Part model, mm, in its own coordinate system. Face numbers are marked on the shaded views. A direction names the side the tool comes from. Round coordinates to 2 decimals unless told otherwise and drop trailing zeros. Loops run counter-clockwise (first coordinate to the right, second up) from the corner with the lowest first, then second, coordinate; pieces in that order, holes last. Notation, with made-up numbers: M 18,29.25 L 57,29.25 A17 ccw 57,44.25 Z; hole C 40.5,34.5 d5. An arc over 180 degrees is marked long. Answer as CSV lines item,"result". Start each with the question number.
Item 1: Which spindle directions (+Z, -Z, +X, -X, +Y, -Y) get a long thin tool onto all of the face, cutting with end or side? Do the marked faces 1 and 2. Say none if no direction does.
Item 2: Band-saw the part on B-B (x = 14.5). Give the cut face in (y, z), and give its area (3 significant figures).
Item 3: Drop flat-ended pins along their axis: pin 1 Ø8 at (y, z) = (0, 0) entering from -X; pin 2 Ø0.8 at (x, y) = (29.5, -25.5) entering from +Z; pin 3 Ø0.8 at (x, y) = (29.5, -49) entering from -Z; pin 4 Ø11 at (y, z) = (-47, -2.5) entering from +X. Give the stop position or say it passes through.
Item 4: Band-saw the part on C-C (x = -2). Give the cut face in (y, z).
Item 5: Wall check: line 1 (X direction, y = -69, z = -3); line 2 (Y direction, x = 17, z = 0); line 3 (X direction, y = -26.5, z = -5.5). Give the ranges that are in metal, low to high.
Item 6: Mould opens along Z. For the marked faces 3, 4, 5 and 6 say: pulls with the +Z half, pulls with the -Z half, needs draft (parallel to the pull), parting line crosses it, or undercut.
```python
from build123d import *

# Parameters (mm, degrees)
SKETCH_1_R          = 4.9
EXTRUDE_1_DEPTH     = 10
EXTRUDE_2_DEPTH     = 20
SKETCH_3_R          = 7.45
EXTRUDE_3_DEPTH     = 31
CHAMFER_1_SIZE      = 2
CUT_EXTRUDE_1_DEPTH = 1
SKETCH_5_R          = 4.9
CUT_EXTRUDE_2_DEPTH = 25
SKETCH_9_R          = 10
EXTRUDE_4_DEPTH     = 1
CHAMFER_2_SIZE      = 1
CHAMFER_4_SIZE      = 1
CHAMFER_5_SIZE      = 1


with BuildPart() as part:
    # 草图1 → 凸台-拉伸1 (new body)
    with BuildSketch(Plane(origin=(0, 0, 0), x_dir=(0, 0, -1), z_dir=(1, 0, 0))):
        Circle(SKETCH_1_R)
    extrude(amount=EXTRUDE_1_DEPTH)

    # 草图2 → 凸台-拉伸2 (add)
    with BuildSketch(Plane(origin=(10, 0, 0), x_dir=(0, 0, -1), z_dir=(1, 0, 0))):
        with BuildLine():
            Line((15, 0), (15, -70))
            ThreePointArc((15, -70), (0, -85), (-15, -70))
            Line((-15, -70), (-15, 0))
            ThreePointArc((-15, 0), (0, 15), (15, 0))
        make_face()
    extrude(amount=EXTRUDE_2_DEPTH)

    # 草图3 → 凸台-拉伸3 (add)
    with BuildSketch(Plane.ZY.offset(-10)):
        with Locations(Location((0, -70, 0), (0, 0, 180))):
            Circle(SKETCH_3_R)
    extrude(amount=EXTRUDE_3_DEPTH)

    # 倒角1
    chamfer_1_edges = [part.edges().sort_by_distance(p)[0] for p in [
        (10, -35, 15),
        (10, -85, 0),
        (30, -35, -15),
        (10, 15, 0),
        (30, -35, 15),
        (30, -85, 0),
        (30, 15, 0),
        (10, -35, -15),
    ]]
    chamfer(chamfer_1_edges, length=CHAMFER_1_SIZE)

    # 草图4 → 切除-拉伸1 (cut)
    with BuildSketch(Plane(origin=(30, 0, 0), x_dir=(0, 0, -1), z_dir=(1, 0, 0))):
        with BuildLine():
            Line((6.835634275, 0), (6.835634275, -70))
            ThreePointArc((6.835634275, -70), (0, -76.835634275), (-6.835634275, -70))
            Line((-6.835634275, -70), (-6.835634275, 0))
            ThreePointArc((-6.835634275, 0), (0, 6.835634275), (6.835634275, 0))
        make_face()
    extrude(amount=-CUT_EXTRUDE_1_DEPTH, mode=Mode.SUBTRACT)

    # 草图5 → 切除-拉伸2 (cut)
    with BuildSketch(Plane.ZY):
        Circle(SKETCH_5_R)
    extrude(amount=-CUT_EXTRUDE_2_DEPTH, mode=Mode.SUBTRACT)

    # 草图9 → 凸台-拉伸4 (add)
    with BuildSketch(Plane.ZY.offset(-10)):
        with Locations(Location((0, -70, 0), (0, 0, 180))):
            Circle(SKETCH_9_R)
    extrude(amount=EXTRUDE_4_DEPTH)

    # 倒角2
    chamfer_2_edges = [part.edges().sort_by_distance(p)[0] for p in [
        (9, -70, 10),
    ]]
    chamfer(chamfer_2_edges, length=CHAMFER_2_SIZE - 0.0001)  # a hair under: the kernel refuses the full size

    # 倒角4
    chamfer_4_edges = [part.edges().sort_by_distance(p)[0] for p in [
        (10, 0, -4.9),
    ]]
    chamfer(chamfer_4_edges, length=CHAMFER_4_SIZE)

    # 倒角5
    chamfer_5_edges = [part.edges().sort_by_distance(p)[0] for p in [
        (-21, -70, 7.45),
    ]]
    chamfer(chamfer_5_edges, length=CHAMFER_5_SIZE)


solid = part.part
```
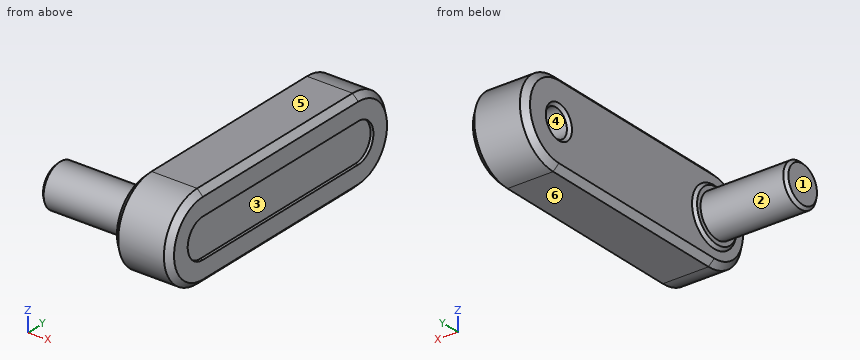
Answer block:
1,face 1,"+Z, -Z, -X, +Y, -Y"
1,face 2,"-X"
2,outline,"M -70,-15 L 0,-15 A15 ccw 0,15 L -70,15 A15 ccw Z; hole C 0,0 d9.8"
2,area,"2,730 mm^2"
3,pin 1,"stops at x = 25"
3,pin 2,"stops at z = 13.9"
3,pin 3,"stops at z = -13.9"
3,pin 4,"stops at x = 30"
4,outline,"C -70,0 d14.9"
5,line 1,"x = -21 to 29"
5,line 2,"y = -85 to -4.9, 4.9 to 15"
5,line 3,"x = 10 to 29"
6,face 3,"undercut"
6,face 4,"undercut"
6,face 5,"pulls with the +Z half"
6,face 6,"pulls with the -Z half"
